Part print with two shaded views. Sizes in mm from the minimum x, y, z corner. A direction names the side the tool comes from. Round coordinates to 2 decimals unless told otherwise and drop trailing zeros. Write each loop counter-clockwise with the first axis right and the second up, starting at its lowest first coordinate (ties: lowest second). Pieces come first, ordered by that corner, then holes. Notation, with made-up numbers: (21.5, -32.75) -> (27.5, -32.75) arc R23 ccw to (27.5, -22.75) -> close; hole circle Ø7 at (-21.75, -13). An arc over 180 degrees is marked (long way). Answer in a Markdown table with one row per item.
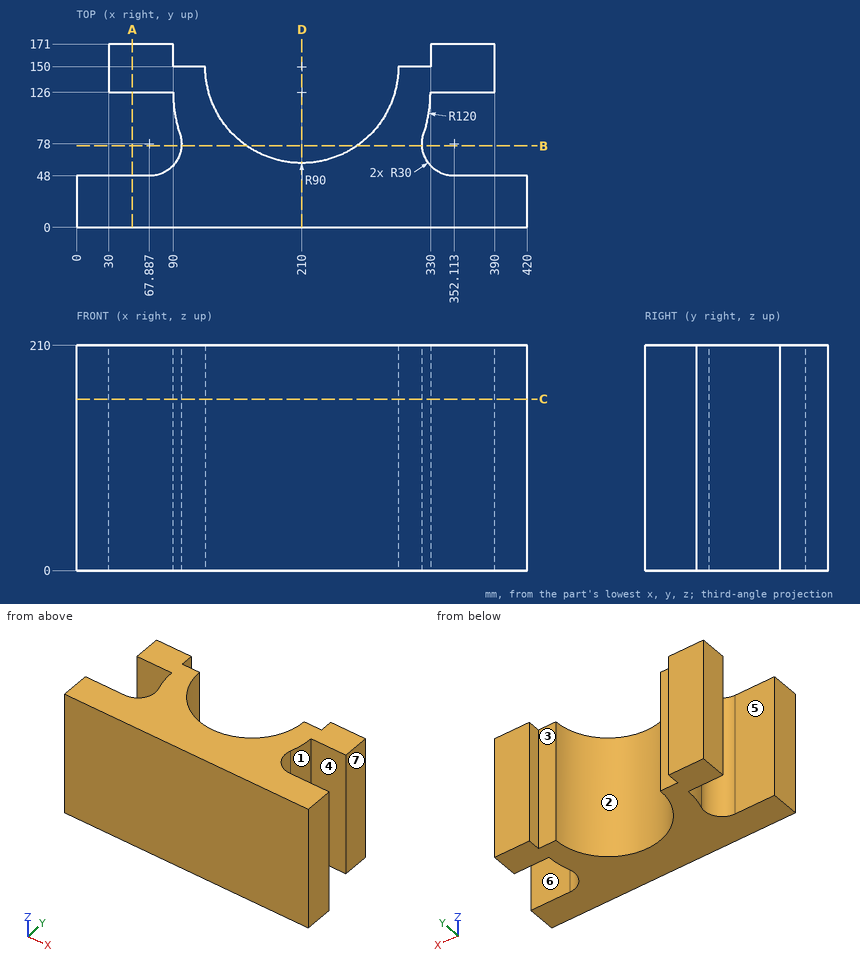
Q1. Saw through at A-A on x = 52. Write the cut outline in (y, z).
A:
| item | result |
|---|---|
| outline | (0, 0) -> (48, 0) -> (48, 210) -> (0, 210) -> close; (126, 0) -> (171, 0) -> (171, 210) -> (126, 210) -> close |
Q2. Saw through at C-C on z = 160. Write the cut outline in (x, y).
A:
| item | result |
|---|---|
| outline | (0, 0) -> (420, 0) -> (420, 48) -> (352.11, 48) arc R30 cw to (323.69, 87.6) arc R120 ccw to (330, 126) -> (390, 126) -> (390, 171) -> (330, 171) -> (330, 150) -> (300, 150) arc R90 cw to (120, 150) -> (90, 150) -> (90, 171) -> (30, 171) -> (30, 126) -> (90, 126) arc R120 ccw to (96.31, 87.6) arc R30 cw to (67.89, 48) -> (0, 48) -> close |
Q3. Saw through at B-B on y = 76. Write the cut outline in (x, z) (1 decimal), plus the area to 3 significant figures.
A:
| item | result |
|---|---|
| outline | (97.8, 0) -> (158.8, 0) -> (158.8, 210) -> (97.8, 210) -> close; (261.2, 0) -> (322.2, 0) -> (322.2, 210) -> (261.2, 210) -> close |
| area | 25,600 mm² |
Q4. Two-plate mould, pull along X, no slides. Class the marked faces 1, 2, 3 and 4: released by +X, released by -X, zero draft, split by the parting line, or undercut.
A:
| item | result |
|---|---|
| face 1 | released by +X |
| face 2 | undercut |
| face 3 | undercut |
| face 4 | zero draft |
Q5. Drop flat-ended pins along their axis: P1, Ø4, axis at y = 141.5, z = 58, coming from the -X side; P2, Ø15, axis at x = 98, z = 59, coming from the +Y side; P3, Ø5, axis at y = 113.5, z = 125, coming from the +X side. Give the stop position or say it passes through.
A:
| item | result |
|---|---|
| P1 | x = 30 |
| P2 | y = 150 |
| P3 | x = 329.58 |
Q6. Saw through at D-D on x = 210. Write the cut outline in (y, z).
A:
| item | result |
|---|---|
| outline | (0, 0) -> (60, 0) -> (60, 210) -> (0, 210) -> close |
Q7. Wall check: line 1 (X direction, y = 152.5, z = 73.5); line 2 (Y direction, x = 385.5, z = 173.5); line 3 (Y direction, x = 76, z = 159). Give the ranges that are in metal, low to high. Write a range as [from, to].
A:
| item | result |
|---|---|
| line 1 | [30, 90], [330, 390] |
| line 2 | [0, 48], [126, 171] |
| line 3 | [0, 49.12], [126, 171] |
Q8. Which spindle directions (+Z, -Z, +X, -X, +Y, -Y) get a long thin tool onto all of the face, cutting with end or side? Do the marked faces 5, 6 and 7. Say none if no direction does.
A:
| item | result |
|---|---|
| face 5 | +Z, -Z, -X |
| face 6 | +Z, -Z, +X |
| face 7 | +Z, -Z, +X, +Y |
